Here's how the part is built. I have some questions about the finished solid (model axes, mm). A direction names the side the tool comes from. Give positions to 0.01 mm unless a question says otherwise; leave off trailing zeros. Loops run counter-clockwise (first coordinate to the right, second up) from the corner with the lowest first, then second, coordinate; pieces in that order, holes last. Notation, with made-up numbers: (-29, 20.25) - (-24, 20.25) arc R8 ccw to (-24, 30.25) - close; hole circle Ø7 at (9, 6.5). An arc over 180 degrees is marked (long way). Use a Markdown table: item, result.
from build123d import *

# Parameters (mm, degrees)
ESQUISSE1_R             = 15
BOSS_EXTRU_1_DEPTH      = 150
ESQUISSE3_OUTSIDE_W     = 92.312
ESQUISSE3_OUTSIDE_H     = 167.312
ESQUISSE3_OUTSIDE_R     = 20
ENL_V_MAT_EXTRU_2_DEPTH = 50


with BuildPart() as part:
    # Esquisse1 → Boss.-Extru.1 (new body)
    with BuildSketch(Plane.XY):
        with BuildLine():
            Line((-10, 52.087121525), (-10, 22.912878475))
            ThreePointArc((-10, 22.912878475), (0, -25), (10, 22.912878475))
            Line((10, 22.912878475), (10, 52.087121525))
            ThreePointArc((10, 52.087121525), (0, 100), (-10, 52.087121525))
        make_face()
        Circle(ESQUISSE1_R, mode=Mode.SUBTRACT)
        with Locations((0, 75)):
            Circle(ESQUISSE1_R, mode=Mode.SUBTRACT)
    extrude(amount=BOSS_EXTRU_1_DEPTH)

    # Esquisse3 outside → Enlèv. mat.-Extru.2 (cut)
    with BuildSketch(Plane.XY.offset(150)):
        with Locations((0, 37.5)):
            Rectangle(ESQUISSE3_OUTSIDE_W, ESQUISSE3_OUTSIDE_H)
        with Locations((0, 75)):
            Circle(ESQUISSE3_OUTSIDE_R, mode=Mode.SUBTRACT)
        Circle(ESQUISSE3_OUTSIDE_R, mode=Mode.SUBTRACT)
    extrude(amount=-ENL_V_MAT_EXTRU_2_DEPTH, mode=Mode.SUBTRACT)


solid = part.part
(1) Suppose I cut it at D-D on x = -12.5. Write out the boundary of the cut face in (y, z).
A:
| item | result |
|---|---|
| outline | (-21.65, 0) - (-8.29, 0) - (-8.29, 150) - (-15.61, 150) - (-15.61, 100) - (-21.65, 100) - close; (8.29, 0) - (21.65, 0) - (21.65, 100) - (15.61, 100) - (15.61, 150) - (8.29, 150) - close; (53.35, 0) - (66.71, 0) - (66.71, 150) - (59.39, 150) - (59.39, 100) - (53.35, 100) - close; (83.29, 0) - (96.65, 0) - (96.65, 100) - (90.61, 100) - (90.61, 150) - (83.29, 150) - close |
(2) Suppose I cut it at C-C on z = 98. Write out the boundary of the cut face in (x, y), plus the area to 3 significant figures.
A:
| item | result |
|---|---|
| outline | (-10, 22.91) arc R25 ccw (long way) to (10, 22.91) - (10, 52.09) arc R25 ccw (long way) to (-10, 52.09) - close; hole circle Ø30 at (0, 0); hole circle Ø30 at (0, 75) |
| area | 3,040 mm2 |
(3) If I drill on line 1 (Y direction, x = 0, z = 63); line 2 (Y direction, x = -3, z = 73.5); line 3 (Y direction, x = -10.5, z = 104), over which ranges is the centre line in solid material (lowest first)?
A:
| item | result |
|---|---|
| line 1 | -25 to -15, 15 to 60, 90 to 100 |
| line 2 | -24.82 to -14.7, 14.7 to 60.3, 89.7 to 99.82 |
| line 3 | -17.02 to -10.71, 10.71 to 17.02, 57.98 to 64.29, 85.71 to 92.02 |
(4) Suppose I cut it at A-A on y = 0. Write out the boundary of the cut face in (x, z), plus the area to 3 significant figures.
A:
| item | result |
|---|---|
| outline | (-25, 0) - (-15, 0) - (-15, 150) - (-20, 150) - (-20, 100) - (-25, 100) - close; (15, 0) - (25, 0) - (25, 100) - (20, 100) - (20, 150) - (15, 150) - close |
| area | 2,500 mm2 |
(5) Suppose I cut it at B-B on x = 0. Write out the boundary of the cut face in (y, z).
A:
| item | result |
|---|---|
| outline | (-25, 0) - (-15, 0) - (-15, 150) - (-20, 150) - (-20, 100) - (-25, 100) - close; (15, 0) - (60, 0) - (60, 150) - (55, 150) - (55, 100) - (20, 100) - (20, 150) - (15, 150) - close; (90, 0) - (100, 0) - (100, 100) - (95, 100) - (95, 150) - (90, 150) - close |
(6) Will these pins go through, and if not, where does the flat tip stop? pin 1 (24 mm diameter, centred on x = 0, y = 75, fed in from -Z); pin 2 (8 mm diameter, centred on x = -3, z = 34, fed in from -Y); pin 3 (1.5 mm diameter, centred on y = 46, z = 72, fed in from -X); pin 4 (12 mm diameter, centred on x = 0.5, z = 66, fed in from +Y).
A:
| item | result |
|---|---|
| pin 1 | through |
| pin 2 | y = -25 |
| pin 3 | x = -10 |
| pin 4 | y = 100 |
(7) We'd pull the mould along Y, two halves only. Please class faces 5 (the face through (-14.985, 0.66, 73.95)), 6 (the face through (0, 38, 0)): pulls with the +Y half, pulls with the -Y half, needs draft (parallel to the pull), parting line crosses it, or undercut.
A:
| item | result |
|---|---|
| face 5 | undercut |
| face 6 | needs draft |
(8) On a 3-axis mill with a long thin cutter (end or side, diameter ignored), from which of +Z, -Z, +X, -X, +Y, -Y can I reach the whole of each face in a straight line? I mean faces 1 (the face through (-10, 38, 49)), 2 (the face through (10, 37, 49)), 3 (the face through (-4.336, 55.476, 125.35)), 4 (the face through (3, 15, 150)). Say none if no direction works.
A:
| item | result |
|---|---|
| face 1 | +Z, -Z, -X |
| face 2 | +Z, -Z, +X |
| face 3 | +Z |
| face 4 | +Z, +X, -X, +Y, -Y |
